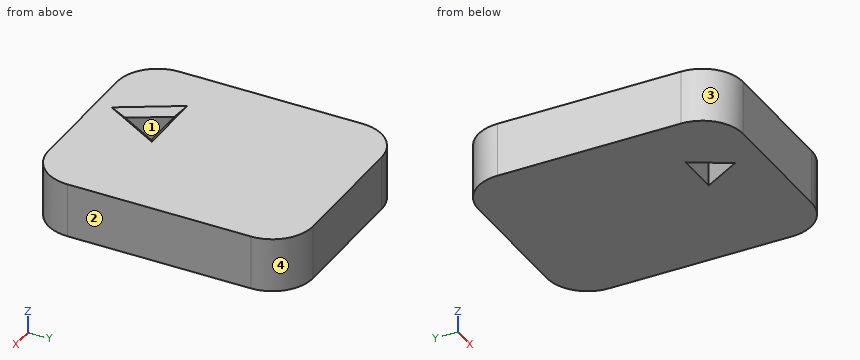
```python
from build123d import *

# Parameters (mm, degrees)
F0_W     = 15.5
F0_H     = 19.5
F1_DEPTH = 4
F3_DEPTH = 4.001
F4_SIZE  = 0.5
F5_R     = 3


with BuildPart() as f1:
    # F0 (on Top) → F1 (new body)
    with BuildSketch(Plane.XY):
        with Locations((-7.75, 9.75)):
            Rectangle(F0_W, F0_H)
    extrude(amount=F1_DEPTH)

    # F2 (on Top) → F3 (cut, through all)
    with BuildSketch(Plane.XY):
        Polygon((-11.202147, 4.925), (-9.6, 2.15), (-7.997853, 4.925), align=None)
    extrude(amount=F3_DEPTH, mode=Mode.SUBTRACT)

    # F4
    f4_edges = [f1.edges().sort_by_distance(p)[0] for p in [
        (-9.6, 4.925, 4),
        (-10.401073, 3.5375, 4),
        (-8.798927, 3.5375, 4),
    ]]
    chamfer(f4_edges, length=F4_SIZE)

    # F5
    f5_edges = [f1.edges().sort_by_distance(p)[0] for p in [
        (-15.5, 0, 2),
        (0, 0, 2),
        (0, 19.5, 2),
        (-15.5, 19.5, 2),
    ]]
    fillet(f5_edges, radius=F5_R)


solid = f1.part
```
Work out the finished part from the listing and answer in its coordinate system (mm). Face numbers are marked on the shaded views. Coordinates: 2 decimals unless noted, no trailing zeros. Loops run counter-clockwise (first coordinate to the right, second up) from the corner with the lowest first, then second, coordinate; pieces in that order, holes last.
1) For a pull along Y with two mould halves and no side action, classify the marked faces 1, 2, 3 and 4 as +Y half, -Y half, draft (parallel to the pull), parting line (faces both ways), or undercut.
Results:
face 1: undercut
face 2: draft
face 3: -Y half
face 4: +Y half
2) Section B-B (x = -10) is taken. Give the vertices of the cut face in (y, z) (3 decimals), plus the area to 3 significant figures.
Results:
outline: (0, 0) - (2.843, 0) - (2.843, 3.5) - (1.843, 4) - (0, 4) - close; (4.925, 0) - (19.5, 0) - (19.5, 4) - (5.425, 4) - (4.925, 3.5) - close
area: 69.3 mm2
3) Consider probe 1 along X at (y, z) = (4.5, 2.9); probe 2 along Y at (x, z) = (-10.25, 3.1) (3 decimals); probe 3 along X at (y, z) = (2.5, 3). Determine where each line is inside the solid, lowest interval first.
Results:
probe 1: x = -15.5 to -10.96, -8.24 to 0
probe 2: y = 0 to 3.276, 4.925 to 19.5
probe 3: x = -15.46 to -9.8, -9.4 to -0.04
4) Section C-C (y = 3.5) is taken. Give the vertices of the cut face in (x, z).
Results:
outline: (-15.5, 0) - (-10.38, 0) - (-10.38, 3.5) - (-10.96, 4) - (-15.5, 4) - close; (-8.82, 0) - (0, 0) - (0, 4) - (-8.24, 4) - (-8.82, 3.5) - close
5) Section D-D (x = -1.75) is taken. Give the vertices of the cut face in (y, z), plus the area to 3 significant figures.
Results:
outline: (0.27, 0) - (19.23, 0) - (19.23, 4) - (0.27, 4) - close
area: 75.8 mm2
6) Section A-A (z = 2.1) is taken. Give the vertices of the cut face in (x, y) (3 decimals), plus the area to 3 significant figures.
Results:
outline: (-15.5, 3) arc R3 ccw to (-12.5, 0) - (-3, 0) arc R3 ccw to (0, 3) - (0, 16.5) arc R3 ccw to (-3, 19.5) - (-12.5, 19.5) arc R3 ccw to (-15.5, 16.5) - close; hole (-11.202, 4.925) - (-9.6, 2.15) - (-7.998, 4.925) - close
area: 290 mm2
